Can you work these out from the drawing? Everything is in mm from the part's minimum corner. Coordinates: 2 decimals unless noted, no trailing zeros. Loops run counter-clockwise (first coordinate to the right, second up) from the corner with the lowest first, then second, coordinate; pieces in that order, holes last. Notation, with made-up numbers: (18, -1.5) - (53, -1.5) arc R35 ccw to (53, 36.5) - close; hole circle Ø5 at (61.25, 51.5). An arc over 180 degrees is marked (long way). Put each result on its own line as item: value. Start each with the question number.
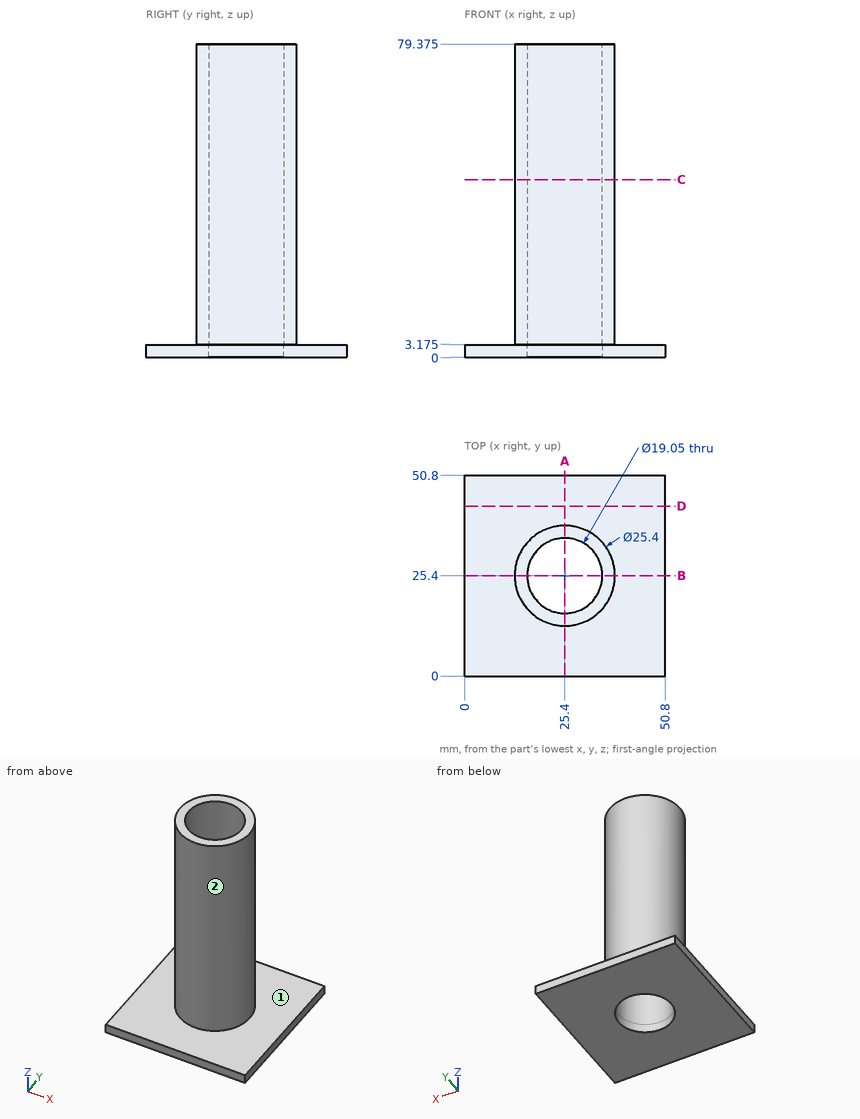
Q1. We'd pull the mould along X, two halves only. Please class the marked faces 1 and 2: released by +X, released by -X, zero draft, split by the parting line, or undercut.
Q2. I want a section at D-D on y = 43. List the corners of the cut face in (x, z) for me (3 decimals), and give its area (3 significant figures).
Q3. I want a section at C-C on z = 45. List the corners of the cut face in (x, y) for me (3 decimals), and give its area (3 significant figures).
Q4. Will these pins go through, and if not, where does the flat tip stop? pin 1 (15 mm diameter, centred on x = 25.4, y = 25.4, fed in from -Z); pin 2 (8 mm diameter, centred on y = 17.5, z = 37, fed in from +X); pin 3 (12 mm diameter, centred on x = 37, y = 7.5, fed in from +Z) (3 decimals); pin 4 (8 mm diameter, centred on y = 30.5, z = 52.5, fed in from +X).
Q5. I want a section at A-A on x = 25.4. List the corners of the cut face in (y, z) for me (3 decimals), and give its area (3 significant figures).
Q6. Please list where these lines run through material, in increasing order: line 1 along Y through (x, z) = (25, 46); line 2 along X through (y, z) = (25, 1). Write a range as [from, to].
Calculated:
1. face 1: zero draft
1. face 2: split by the parting line
2. outline: (0, 0) - (50.8, 0) - (50.8, 3.175) - (0, 3.175) - close
2. area: 161 mm2
3. outline: circle Ø25.4 at (25.4, 25.4); hole circle Ø19.05 at (25.4, 25.4)
3. area: 222 mm2
4. pin 1: through
4. pin 2: x = 37.49
4. pin 3: z = 3.175
4. pin 4: x = 38.05
5. outline: (0, 0) - (15.875, 0) - (15.875, 79.375) - (12.7, 79.375) - (12.7, 3.175) - (0, 3.175) - close; (34.925, 0) - (50.8, 0) - (50.8, 3.175) - (38.1, 3.175) - (38.1, 79.375) - (34.925, 79.375) - close
5. area: 585 mm2
6. line 1: [12.71, 15.88], [34.92, 38.09]
6. line 2: [0, 15.88], [34.92, 50.8]
